```python
from build123d import *

# Parameters (mm, degrees)
EXTRUDE_1_DEPTH     = 14.45
SKETCH_2_R          = 1.5
CUT_EXTRUDE_1_DEPTH = 3
CHAMFER_1_SIZE      = 0.5


with BuildPart() as part:
    # 草图1 → 凸台-拉伸1 (new, symmetric)
    with BuildSketch(Plane.XY):
        Polygon((-4.5, 0), (-4.5, -4.5), (-10, -4.5), (-10, 3.5), (10, 3.5), (10, -4.5), (4.5, -4.5), (4.5, 0), align=None)
    extrude(amount=EXTRUDE_1_DEPTH, both=True)

    # 草图2 → 切除-拉伸1 (cut)
    with BuildSketch(Plane(origin=(0, 3.5, 0), x_dir=(1, 0, 0), z_dir=(0, 1, 0))):
        with Locations(Location((-7.5, 5, 0), (0, 0, 180))):
            Circle(SKETCH_2_R)
        with Locations(Location((7.5, 5, 0), (0, 0, 180))):
            Circle(SKETCH_2_R)
        with Locations(Location((-7.5, -5, 0), (0, 0, 180))):
            Circle(SKETCH_2_R)
        with Locations(Location((7.5, -5, 0), (0, 0, 180))):
            Circle(SKETCH_2_R)
    extrude(amount=-CUT_EXTRUDE_1_DEPTH, mode=Mode.SUBTRACT)

    # 倒角1
    chamfer_1_edges = [part.edges().sort_by_distance(p)[0] for p in [
        (-4.5, -4.5, 0),
        (-10, -4.5, 0),
        (-10, 3.5, 0),
        (10, 3.5, 0),
        (10, -4.5, 0),
        (4.5, -4.5, 0),
    ]]
    chamfer(chamfer_1_edges, length=CHAMFER_1_SIZE)


solid = part.part
```
Read the model definition and answer for the solid it produces. Units are mm, in the model's axes. A direction names the side the tool comes from. Coordinates: 2 decimals unless noted, no trailing zeros. Loops run counter-clockwise (first coordinate to the right, second up) from the corner with the lowest first, then second, coordinate; pieces in that order, holes last. Notation, with made-up numbers: (57, 33) - (110, 33) arc R21 cw to (110, 67) - close; hole circle Ø5 at (-23.75, 3). An arc over 180 degrees is marked (long way). Answer in a Markdown table with one row per item.
1. Find section C-C, the plane x = -7.5. Write down the section's boundary in (y, z), then the cut area to 3 significant figures.
Conclusion:
| item | result |
|---|---|
| outline | (-4.5, -14.45) - (3.5, -14.45) - (3.5, -6.5) - (0.5, -6.5) - (0.5, -3.5) - (3.5, -3.5) - (3.5, 3.5) - (0.5, 3.5) - (0.5, 6.5) - (3.5, 6.5) - (3.5, 14.45) - (-4.5, 14.45) - close |
| area | 213 mm² |
2. Given pin 1 (2.5 mm diameter, centred on x = 7.5, z = -5, fed in from +Y); pin 2 (7 mm diameter, centred on x = -0.5, z = -2, fed in from -Y); pin 3 (3.5 mm diameter, centred on x = 7, z = -5, fed in from +Y), each flat-ended and moving along its own axis, determine where each tip first touches the part or whether it passes through.
Conclusion:
| item | result |
|---|---|
| pin 1 | stops at y = 0.5 |
| pin 2 | stops at y = 0 |
| pin 3 | stops at y = 3.5 |
3. Determine the mould class of faces 4 (the face through (0.1, 0.4, -14.45)), 5 (the face through (-4.5, -2, 0)), 6 (the face through (-7, 0.5, 5)), 7 (the face through (-7, 0.5, -5)) for opening direction Z: +Z half, -Z half, draft (parallel to the pull), parting line (faces both ways), or undercut.
Conclusion:
| item | result |
|---|---|
| face 4 | -Z half |
| face 5 | draft |
| face 6 | undercut |
| face 7 | undercut |
4. Find section B-B, the plane z = -11.5. Write down the section's boundary in (x, y), then the cut area to 3 significant figures.
Conclusion:
| item | result |
|---|---|
| outline | (-10, -4) - (-9.5, -4.5) - (-5, -4.5) - (-4.5, -4) - (-4.5, 0) - (4.5, 0) - (4.5, -4) - (5, -4.5) - (9.5, -4.5) - (10, -4) - (10, 3) - (9.5, 3.5) - (-9.5, 3.5) - (-10, 3) - close |
| area | 119 mm² |
5. Which of the six approach directions +Z, -Z, +X, -X, +Y, -Y give full straight-line access (tool end or side, diameter ignored) to faces 1 (the face through (-6, 2, -5)), 2 (the face through (0, 3.5, 0)), 3 (the face through (0, 0, 0))?
Conclusion:
| item | result |
|---|---|
| face 1 | +Y |
| face 2 | +Z, -Z, +X, -X, +Y |
| face 3 | +Z, -Z, -Y |
6. Straight lines are drawn through the part: line 1 (Z direction, x = 7.5, y = 1.6); line 2 (X direction, y = -0.75, z = -3.5); line 3 (X direction, y = 1.25, z = -6). For each, find the intervals that lie inside material, in ascending order.
Conclusion:
| item | result |
|---|---|
| line 1 | z = -14.45 to -6.5, -3.5 to 3.5, 6.5 to 14.45 |
| line 2 | x = -10 to -4.5, 4.5 to 10 |
| line 3 | x = -10 to -8.62, -6.38 to 6.38, 8.62 to 10 |
7. Find section A-A, the plane y = -1. Write down the section's boundary in (x, z).
Conclusion:
| item | result |
|---|---|
| outline | (-10, -14.45) - (-4.5, -14.45) - (-4.5, 14.45) - (-10, 14.45) - close; (4.5, -14.45) - (10, -14.45) - (10, 14.45) - (4.5, 14.45) - close |
8. Find section D-D, the plane y = 2.5. Write down the section's boundary in (x, z).
Conclusion:
| item | result |
|---|---|
| outline | (-10, -14.45) - (10, -14.45) - (10, 14.45) - (-10, 14.45) - close; hole circle Ø3 at (-7.5, -5); hole circle Ø3 at (-7.5, 5); hole circle Ø3 at (7.5, -5); hole circle Ø3 at (7.5, 5) |
